Here's the drawing with two shaded views (mm, measured from the low corner). I have some questions. A direction names the side the tool comes from. Coordinates: 2 decimals unless noted, no trailing zeros. Loops run counter-clockwise (first coordinate to the right, second up) from the corner with the lowest first, then second, coordinate; pieces in that order, holes last. Notation, with made-up numbers: M 35,57 L 87,57 A19 cw 87,63 Z; hole C 78.5,53 d10. An arc over 180 degrees is marked long. Return JSON: item names as keys, results as strings. Group by question number.
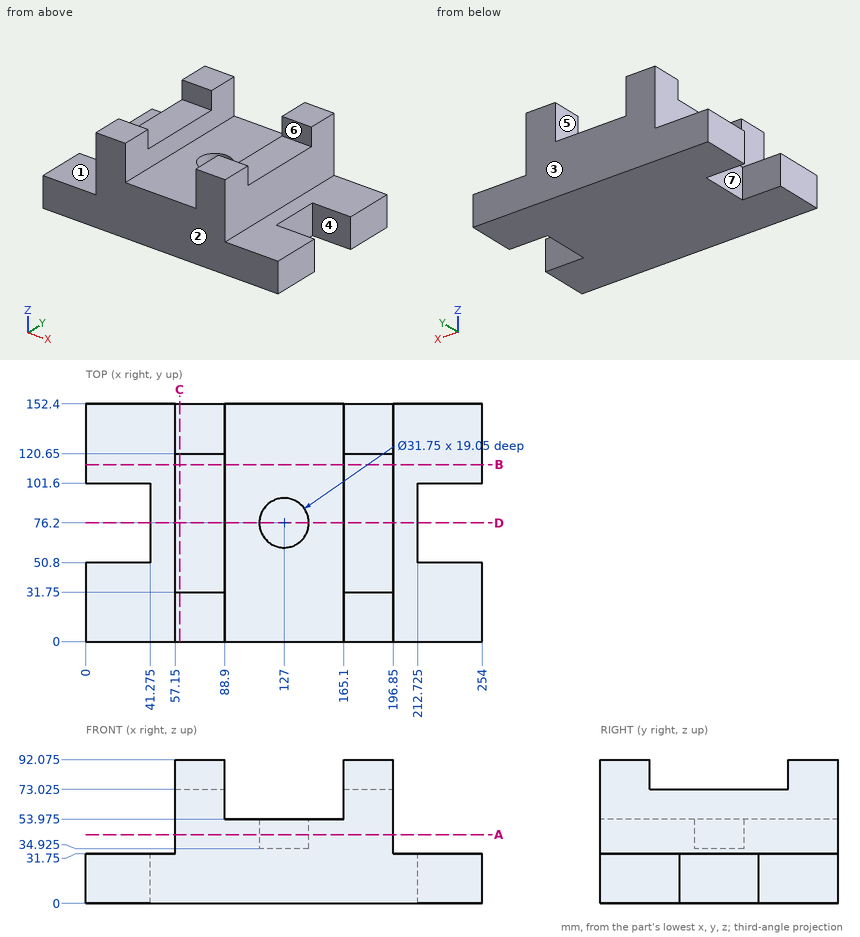
(1) For the marked faces 5, 6 and 7, which set-ups out of +Z, -Z, +X, -X, +Y, -Y let a thin tool reach every point of the face, with its end or its side?
(2) Will these pins go through, and if not, where does the flat tip stop? P1, Ø3, axis at x = 123, z = 26, coming from the -Y side; P2, Ø1, axis at y = 40, z = 58.5, coming from the -X side; P3, Ø23, axis at x = 131, y = 108.5, coming from the +Z side (3 decimals); P4, Ø9.5, axis at x = 130.5, y = 79.5, coming from the +Z side (3 decimals).
(3) If I drill on L1, parallel to Y at x = 127, z = 45 (3 decimals); L2, parallel to X at y = 76, z = 42; L3, parallel to X at y = 145.5, z = 74, over which ranges is the centre line in solid material (lowest first)? Write a range as [from, to].
(4) Imagine slicing it at D-D, the plane y = 76.2. Write out the boundary of the cut face in (x, z) (3 decimals).
(5) Imagine slicing it at C-C, the plane x = 60. Write out the boundary of the cut face in (y, z) (3 decimals), then the cut area to 3 significant figures.
(6) Imagine slicing it at B-B, the plane y = 113.5. Write out the boundary of the cut face in (x, z) (3 decimals), then the cut area to 3 significant figures.
(7) We'd pull the mould along Y, two halves only. Please class the marked faces 1, 2, 3 and 4: +Y half, -Y half, draft (parallel to the pull), parting line (faces both ways), or undercut.
(8) Imagine slicing it at A-A, the plane z = 44. Write out the boundary of the cut face in (x, y) (3 decimals), then the cut area to 3 significant figures.
Checks:
{
 "1": {"face 5": "+Z, +Y, -Y", "face 6": "+Z, +X, -X", "face 7": "+Z, -Z, -X"},
 "2": {"P1": "y = 0", "P2": "x = 57.15", "P3": "z = 53.975", "P4": "z = 34.925"},
 "3": {"L1": "[0, 60.325], [92.075, 152.4]", "L2": "[57.15, 111.13], [142.87, 196.85]", "L3": "[57.15, 88.9], [165.1, 196.85]"},
 "4": {"outline": "M 41.275,0 L 212.725,0 L 212.725,31.75 L 196.85,31.75 L 196.85,73.025 L 165.1,73.025 L 165.1,53.975 L 142.875,53.975 L 142.875,34.925 L 111.125,34.925 L 111.125,53.975 L 88.9,53.975 L 88.9,73.025 L 57.15,73.025 L 57.15,31.75 L 41.275,31.75 Z"},
 "5": {"outline": "M 0,0 L 152.4,0 L 152.4,92.075 L 120.65,92.075 L 120.65,73.025 L 31.75,73.025 L 31.75,92.075 L 0,92.075 Z", "area": "12,300 mm²"},
 "6": {"outline": "M 0,0 L 254,0 L 254,31.75 L 196.85,31.75 L 196.85,73.025 L 165.1,73.025 L 165.1,53.975 L 88.9,53.975 L 88.9,73.025 L 57.15,73.025 L 57.15,31.75 L 0,31.75 Z", "area": "12,400 mm²"},
 "7": {"face 1": "draft", "face 2": "-Y half", "face 3": "+Y half", "face 4": "undercut"},
 "8": {"outline": "M 57.15,0 L 196.85,0 L 196.85,152.4 L 57.15,152.4 Z; hole C 127,76.2 d31.75", "area": "20,500 mm²"}
}
